Check sheet for the modelled part. Datum: model origin and axes. Units: mm. Coordinates: 2 decimals unless noted, no trailing zeros. Loops run counter-clockwise (first coordinate to the right, second up) from the corner with the lowest first, then second, coordinate; pieces in that order, holes last. Notation, with made-up numbers: M -9,74.25 L 7,74.25 A17 cw 7,105.25 Z; hole C 67.25,14 d6. An arc over 180 degrees is marked long. Return JSON: item names as keys, results as strings.
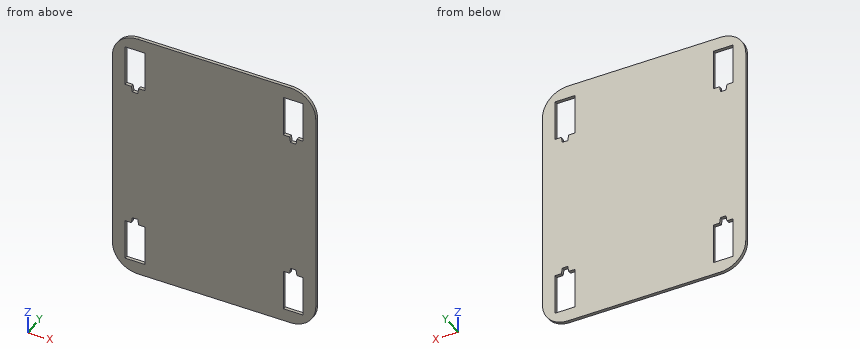
from build123d import *

# Parameters (mm, degrees)
SKETCH1_W               = 203.2
SKETCH1_H               = 254
BOSS_EXTRUDE1_DEPTH     = 3.175
FILLET1_R               = 25.4
SKETCH2_W               = 19.6508
SKETCH2_H               = 40.550799923
CUT_EXTRUDE1_DEPTH      = 163.67034341
CUT_EXTRUDE2_DEPTH      = 163.67034341
MIRROR2_COPY_1_SKETCH_W = 19.6508
MIRROR2_COPY_1_SKETCH_H = 40.550799923
MIRROR2_COPY_1_DEPTH    = 163.67034341
MIRROR2_COPY_2_DEPTH    = 163.67034341


with BuildPart() as part:
    # Sketch1 → Boss-Extrude1 (new body)
    with BuildSketch(Plane(origin=(0, 0, 0), x_dir=(1, 0, 0), z_dir=(0, 1, 0))):
        Rectangle(SKETCH1_W, SKETCH1_H)
    extrude(amount=BOSS_EXTRUDE1_DEPTH)

    # Fillet1
    fillet1_edges = [part.edges().sort_by_distance(p)[0] for p in [
        (101.6, 1.5875, 127),
        (-101.6, 1.5875, 127),
        (-101.6, 1.5875, -127),
        (101.6, 1.5875, -127),
    ]]
    fillet(fillet1_edges, radius=FILLET1_R)

    # Sketch2 → Cut-Extrude1 (cut, through all)
    with BuildSketch(Plane(origin=(0, 3.175, 0), x_dir=(1, 0, 0), z_dir=(0, 1, 0))):
        with Locations((-79.1, 94.050000013)):
            Rectangle(SKETCH2_W, SKETCH2_H)
    cut_extrude1 = extrude(amount=-CUT_EXTRUDE1_DEPTH, mode=Mode.SUBTRACT)

    # Sketch3 → Cut-Extrude2 (cut, through all)
    with BuildSketch(Plane.XZ):
        Polygon((-82.775820479, -73.774600051), (-81.815035673, -68.053121226), (-76.384964327, -68.053121226), (-75.424179521, -73.774600051), align=None)
    cut_extrude2 = extrude(amount=-CUT_EXTRUDE2_DEPTH, mode=Mode.SUBTRACT)

    # Mirror1: Cut-Extrude1, Cut-Extrude2 across plane
    add(cut_extrude1.mirror(Plane(origin=(0, 0, 0), x_dir=(0, 0, 1), z_dir=(1, 0, 0))), mode=Mode.SUBTRACT)
    add(cut_extrude2.mirror(Plane(origin=(0, 0, 0), x_dir=(0, 0, 1), z_dir=(1, 0, 0))), mode=Mode.SUBTRACT)

    # Mirror2: Cut-Extrude1, Cut-Extrude2 across plane
    add(cut_extrude1.mirror(Plane.XY), mode=Mode.SUBTRACT)
    add(cut_extrude2.mirror(Plane.XY), mode=Mode.SUBTRACT)

    # Mirror2 copy 1 sketch → Mirror2 copy 1 (cut, through all)
    with BuildSketch(Plane(origin=(0, 3.175, 0), x_dir=(-1, 0, 0), z_dir=(0, 1, 0))):
        with Locations((-79.1, 94.050000013)):
            Rectangle(MIRROR2_COPY_1_SKETCH_W, MIRROR2_COPY_1_SKETCH_H)
    extrude(amount=-MIRROR2_COPY_1_DEPTH, mode=Mode.SUBTRACT)

    # Mirror2 copy 2 sketch → Mirror2 copy 2 (cut, through all)
    with BuildSketch(Plane(origin=(0, 0, 0), x_dir=(-1, 0, 0), z_dir=(0, -1, 0))):
        Polygon((-82.775820479, -73.774600051), (-81.815035673, -68.053121226), (-76.384964327, -68.053121226), (-75.424179521, -73.774600051), align=None)
    extrude(amount=-MIRROR2_COPY_2_DEPTH, mode=Mode.SUBTRACT)


solid = part.part
1) Section check B-B on y = 1.2. Count the separate pieces of the cut face and the enclosed holes in it, then the cut area to 3 significant figures.
Answers:
{"separate pieces": "1", "enclosed holes": "4", "area": "47,700 mm²"}
2) Scan lines: line 1 along X through (y, z) = (2.75, -95.5); line 2 along X through (y, z) = (2.65, -107); line 3 along Z through (x, y) = (81.5, 0.25). Record each from-to range of solid material in increasing order. Write a range as [from, to].
Answers:
{"line 1": "[-101.6, -88.93], [-69.27, 69.27], [88.93, 101.6]", "line 2": "[-101.02, -88.93], [-69.27, 69.27], [88.93, 101.02]", "line 3": "[-126.44, -114.33], [-68.05, 68.05], [114.33, 126.44]"}
3) Section check A-A on z = -85. Record the cut outline in (x, y) (3 decimals), then the cut area to 3 significant figures.
Answers:
{"outline": "M -101.6,0 L -88.925,0 L -88.925,3.175 L -101.6,3.175 Z; M -69.275,0 L 69.275,0 L 69.275,3.175 L -69.275,3.175 Z; M 88.925,0 L 101.6,0 L 101.6,3.175 L 88.925,3.175 Z", "area": "520 mm²"}
4) Go/stop test with flat-tipped pins: pin 1 Ø1 at (x, y) = (-80, 1) entering from -Z; pin 2 Ø1 at (x, y) = (78.5, 1.5) entering from -Z. Record where each tip stops, or that it passes through.
Answers:
{"pin 1": "z = -126.78", "pin 2": "z = -126.94"}
